Could you check a few things on this model? Use its own coordinates, in mm. Coordinates: 2 decimals unless noted, no trailing zeros. Write each loop counter-clockwise with the first axis right and the second up, starting at its lowest first coordinate (ties: lowest second). Pieces come first, ordered by that corner, then holes.
```python
from build123d import *

# Parameters (mm, degrees)
BOSS_EXTRUDE1_DEPTH = 3
FILLET1_R           = 10
FILLET2_R           = 1.5


with BuildPart() as part:
    # Sketch1 → Boss-Extrude1 (new body)
    with BuildSketch(Plane(origin=(0, 0, 0), x_dir=(1, 0, 0), z_dir=(0, 1, 0))):
        Polygon((0, 0), (100, 0), (100, 50), (80, 50), align=None)
    extrude(amount=BOSS_EXTRUDE1_DEPTH)

    # Fillet1
    fillet1_edges = [part.edges().sort_by_distance(p)[0] for p in [
        (80, 1.5, -50),
    ]]
    fillet(fillet1_edges, radius=FILLET1_R)

    # Fillet2
    fillet2_edges = [part.edges().sort_by_distance(p)[0] for p in [
        (91.433981132, 0, -50),
        (80.111137134, 0, -49.612487462),
        (91.433981132, 3, -50),
        (80.111137134, 3, -49.612487462),
        (100, 3, -25),
        (100, 0, -25),
        (38.783986432, 0, -24.23999152),
        (38.783986432, 3, -24.23999152),
    ]]
    fillet(fillet2_edges, radius=FILLET2_R - 0.0001)  # a hair under: the kernel refuses the full size


solid = part.part
```
1. For pin 1 (1.5 mm diameter, centred on y = 1, z = -29.5, fed in from +X), with a flat end and sliding along its axis, tell me the tip position at first contact or that it passes through.
Verdict:
pin 1: stops at x = 100
2. Please list where these lines run through material, in increasing order: line 1 along X through (y, z) = (1.65, -2.5); line 2 along X through (y, z) = (0.4, -2); line 3 along Z through (x, y) = (13, 2.3).
Verdict:
line 1: x = 4.01 to 99.99
line 2: x = 4.11 to 99.52
line 3: z = -7.85 to 0
3. I want a section at A-A on y = 2.4. Please give me the cut outline in (x, z).
Verdict:
outline: (0.57, 0) - (77.73, -48.23) arc R9.7 ccw to (82.87, -49.7) - (99.7, -49.7) - (99.7, 0) - close
